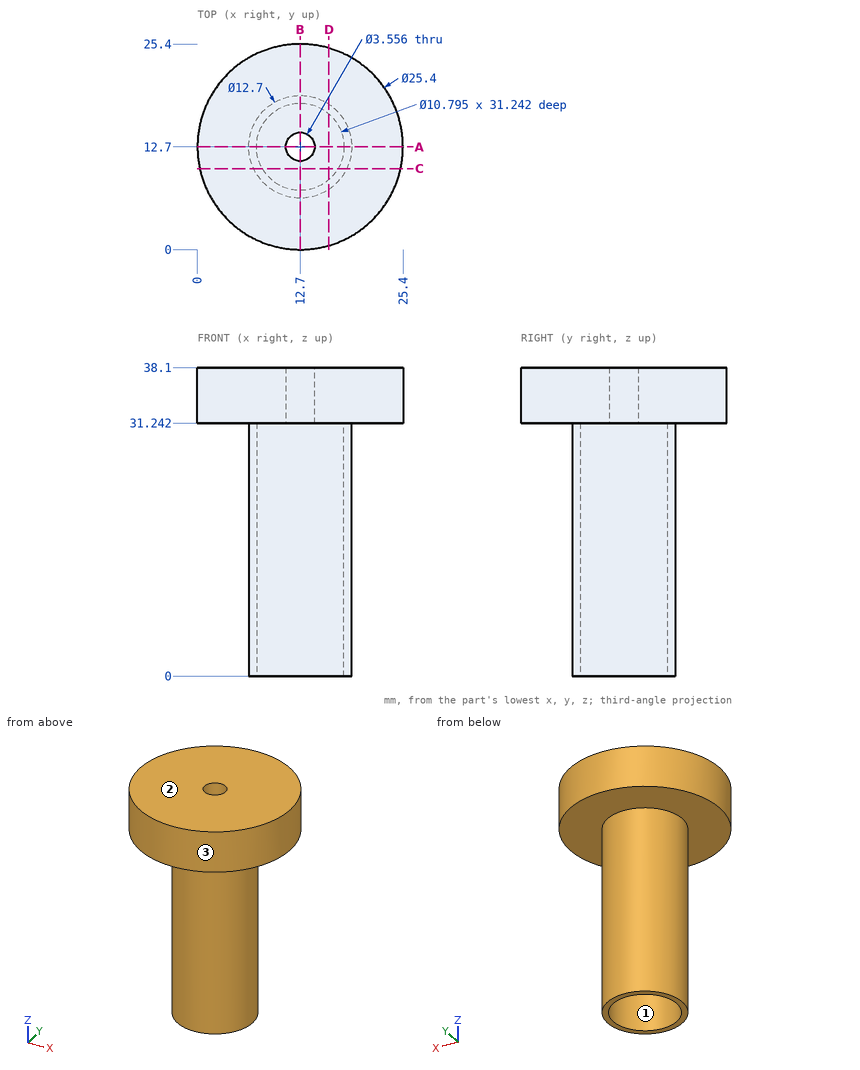
Can you work these out from the drawing? Everything is in mm from the part's minimum corner. Give positions to 0.01 mm unless a question says otherwise; leave off trailing zeros. Order: outer loops, then holes, each group sorted by start corner. A loop starts at its lowest first (then second) coordinate and runs counter-clockwise, first axis right, second up.
Item 1: If we section it at C-C, the plane y = 10: Write out the boundary of the cut face in (x, z), plus the area to 3 significant figures.
Item 2: I need wall thicknesses on line 1 (Y direction, x = 12.7, z = 35); line 2 (X direction, y = 12.7, z = 22). Which ranges of each line are inside material? Lowest first, please.
Item 3: If we section it at D-D, the plane x = 16.25: Write out the boundary of the cut face in (y, z).
Item 4: If we section it at A-A, the plane y = 12.7: Write out the boundary of the cut face in (x, z), plus the area to 3 significant figures.
Item 5: If we mould it in two halves opening along Y, with no side actions, what happens to the marked faces 1, 2 and 3? For each: pulls with the +Y half, pulls with the -Y half, needs draft (parallel to the pull), parting line crosses it, or undercut.
Item 6: I'm going to push flat-ended pins straight in: pin 1 (3 mm diameter, centred on y = 20.5, z = 33.5, fed in from +X); pin 2 (3 mm diameter, centred on y = 19.5, z = 32, fed in from +X); pin 3 (6 mm diameter, centred on y = 7.5, z = 32, fed in from -X). Where does each tip first touch, or does it pass through?
Values:
1. outline: (0.29, 31.24) - (6.95, 31.24) - (6.95, 0) - (8.03, 0) - (8.03, 31.24) - (17.37, 31.24) - (17.37, 0) - (18.45, 0) - (18.45, 31.24) - (25.11, 31.24) - (25.11, 38.1) - (0.29, 38.1) - close
1. area: 237 mm2
2. line 1: y = 0 to 10.92, 14.48 to 25.4
2. line 2: x = 6.35 to 7.3, 18.1 to 19.05
3. outline: (0.51, 31.24) - (7.44, 31.24) - (7.44, 0) - (8.63, 0) - (8.63, 31.24) - (16.77, 31.24) - (16.77, 0) - (17.96, 0) - (17.96, 31.24) - (24.89, 31.24) - (24.89, 38.1) - (0.51, 38.1) - close
4. outline: (0, 31.24) - (6.35, 31.24) - (6.35, 0) - (7.3, 0) - (7.3, 31.24) - (10.92, 31.24) - (10.92, 38.1) - (0, 38.1) - close; (14.48, 31.24) - (18.1, 31.24) - (18.1, 0) - (19.05, 0) - (19.05, 31.24) - (25.4, 31.24) - (25.4, 38.1) - (14.48, 38.1) - close
4. area: 209 mm2
5. face 1: undercut
5. face 2: needs draft
5. face 3: parting line crosses it
6. pin 1: stops at x = 23.73
6. pin 2: stops at x = 24.24
6. pin 3: stops at x = 0.19
